Could you check a few things on this model? Use its own coordinates, in mm. A direction names the side the tool comes from. Round coordinates to 2 decimals unless told otherwise and drop trailing zeros. Loops run counter-clockwise (first coordinate to the right, second up) from the corner with the lowest first, then second, coordinate; pieces in that order, holes last. Notation, with made-up numbers: (82, -29.5) -> (131, -29.5) arc R30 cw to (131, 7.5) -> close; hole circle Ø5 at (-34.5, 82). An arc over 180 degrees is marked (long way). Write each question's results on one line, items separated by ' | '. Start each with the question number.
1) Imagine slicing it at B-B, the plane x = 0. List the corners of the cut face in (y, z) for me.
2) Which directions (+Z, -Z, +X, -X, +Y, -Y) give clear straight access to the entire face, cutting with the end or side of a thin tool? Please do faces 1 (the flat face through (10, -1, 0.6)), 2 (the flat face through (6, 0, 2)).
3) If I drill on probe 1 along Z at (x, y) = (6.25, -1.7); probe 2 along Z at (x, y) = (6.5, 0.4); probe 3 along Y at (x, z) = (6.25, -2.05), over which ranges is the centre line in solid material (lowest first)?
4) Imagine slicing it at C-C, the plane y = -0.4. Give the number of separate pieces and of enclosed holes in the cut face, plus the area to 3 significant figures.
5) For P1, Ø2, axis at x = 8.5, y = -0.5, coming from the -Z side; P2, Ø0.6, axis at x = 0, z = 1, coming from the -Y side; P3, Ø0.9, axis at x = 10, z = 1, coming from the -Y side, each with a flat end and sliding along its axis, tell me the tip position at first contact or that it passes through.
6) Imagine slicing it at D-D, the plane y = 0.75. List the corners of the cut face in (x, z) for me, plus the area to 3 significant figures.
7) Imagine slicing it at A-A, the plane z = -1.8. List the corners of the cut face in (x, y) for me, plus the area to 3 significant figures.
8) We'd pull the mould along Z, two halves only. Please class faces 3 (the flat face through (6, 0, 0)), 4 (the flat face through (8, -1, 1.4)), 5 (the flat face through (2, -1, 1.4)), 6 (the flat face through (13, 0, 1)): pulls with the +Z half, pulls with the -Z half, needs draft (parallel to the pull), parting line crosses it, or undercut.
from build123d import *

# Parameters (mm, degrees)
SKETCH1_W                  = 2
SKETCH1_H                  = 4.5
BOSS_EXTRUDE1_DEPTH        = 2
SKETCH2_W                  = 0.8
SKETCH2_H                  = 0.8
CUT_EXTRUDE1_DEPTH         = 2.8
CHAMFER1_SIZE              = 0.2
SKETCH3_W                  = 3.5
SKETCH3_H                  = 0.2
BOSS_EXTRUDE2_DEPTH        = 0.3
LPATTERN1_COUNT            = 7
LPATTERN1_PITCH            = 2
CHAMFER1_OF_LPATTERN1_SIZE = 0.2


with BuildPart() as part:
    # Sketch1 → Boss-Extrude1 (new body)
    with BuildSketch(Plane.XY):
        Rectangle(SKETCH1_W, SKETCH1_H)
    boss_extrude1 = extrude(amount=BOSS_EXTRUDE1_DEPTH)

    # Sketch2 → Cut-Extrude1 (cut)
    with BuildSketch(Plane.XZ.offset(2.25)):
        with Locations((0, 1)):
            Rectangle(SKETCH2_W, SKETCH2_H)
    cut_extrude1 = extrude(amount=-CUT_EXTRUDE1_DEPTH, mode=Mode.SUBTRACT)

    # Chamfer1
    chamfer1_edges = [part.edges().sort_by_distance(p)[0] for p in [
        (0.4, -2.25, 1),
        (0, -2.25, 1.4),
        (-0.4, -2.25, 1),
        (0, -2.25, 0.6),
    ]]
    chamfer(chamfer1_edges, length=CHAMFER1_SIZE)

    # Sketch3 → Boss-Extrude2 (add, symmetric)
    with BuildSketch(Plane(origin=(0, 0, 0), x_dir=(0, 0, -1), z_dir=(1, 0, 0))):
        with Locations((0.75, 2.35)):
            Rectangle(SKETCH3_W, SKETCH3_H)
    boss_extrude2 = extrude(amount=BOSS_EXTRUDE2_DEPTH, both=True)

    # LPattern1: Boss-Extrude1, Cut-Extrude1, Boss-Extrude2 ×7
    with Locations(*[(i * LPATTERN1_PITCH, 0, 0) for i in range(1, LPATTERN1_COUNT)]):
        add(boss_extrude1)
        add(cut_extrude1, mode=Mode.SUBTRACT)
        add(boss_extrude2)

    # Chamfer1 of LPattern1
    chamfer1_of_lpattern1_edges = [part.edges().sort_by_distance(p)[0] for p in [
        (2.4, -2.25, 1),
        (2, -2.25, 1.4),
        (1.6, -2.25, 1),
        (2, -2.25, 0.6),
        (4.4, -2.25, 1),
        (4, -2.25, 1.4),
        (3.6, -2.25, 1),
        (4, -2.25, 0.6),
        (6.4, -2.25, 1),
        (6, -2.25, 1.4),
        (5.6, -2.25, 1),
        (6, -2.25, 0.6),
        (8.4, -2.25, 1),
        (8, -2.25, 1.4),
        (7.6, -2.25, 1),
        (8, -2.25, 0.6),
        (10.4, -2.25, 1),
        (10, -2.25, 1.4),
        (9.6, -2.25, 1),
        (10, -2.25, 0.6),
        (12.4, -2.25, 1),
        (12, -2.25, 1.4),
        (11.6, -2.25, 1),
        (12, -2.25, 0.6),
    ]]
    chamfer(chamfer1_of_lpattern1_edges, length=CHAMFER1_OF_LPATTERN1_SIZE)


solid = part.part
Checked values:
1) outline: (-2.25, 0) -> (2.25, 0) -> (2.25, -2.5) -> (2.45, -2.5) -> (2.45, 1) -> (2.25, 1) -> (2.25, 2) -> (-2.25, 2) -> (-2.25, 1.6) -> (-2.05, 1.4) -> (0.55, 1.4) -> (0.55, 0.6) -> (-2.05, 0.6) -> (-2.25, 0.4) -> close
2) face 1: -Y | face 2: +Z, +X, -X, +Y, -Y
3) probe 1: 0 to 0.6, 1.4 to 2 | probe 2: 0 to 2 | probe 3: 2.25 to 2.45
4) separate pieces: 1 | enclosed holes: 7 | area: 23.5 mm^2
5) P1: z = 0 | P2: y = 0.55 | P3: y = -2.1
6) outline: (-1, 0) -> (13, 0) -> (13, 2) -> (-1, 2) -> close | area: 28.0 mm^2
7) outline: (-0.3, 2.25) -> (0.3, 2.25) -> (0.3, 2.45) -> (-0.3, 2.45) -> close; (1.7, 2.25) -> (2.3, 2.25) -> (2.3, 2.45) -> (1.7, 2.45) -> close; (3.7, 2.25) -> (4.3, 2.25) -> (4.3, 2.45) -> (3.7, 2.45) -> close; (5.7, 2.25) -> (6.3, 2.25) -> (6.3, 2.45) -> (5.7, 2.45) -> close; (7.7, 2.25) -> (8.3, 2.25) -> (8.3, 2.45) -> (7.7, 2.45) -> close; (9.7, 2.25) -> (10.3, 2.25) -> (10.3, 2.45) -> (9.7, 2.45) -> close; (11.7, 2.25) -> (12.3, 2.25) -> (12.3, 2.45) -> (11.7, 2.45) -> close | area: 0.840 mm^2
8) face 3: pulls with the -Z half | face 4: undercut | face 5: undercut | face 6: needs draft
